from build123d import *

# Parameters (mm, degrees)
SKETCH1_R           = 9
BOSS_EXTRUDE1_DEPTH = 36
BOSS_EXTRUDE2_DEPTH = 12
SKETCH3_W           = 60
SKETCH3_H           = 72
BOSS_EXTRUDE3_DEPTH = 12
SKETCH4_W           = 13
SKETCH4_H           = 12
BOSS_EXTRUDE4_DEPTH = 60
BOSS_EXTRUDE5_DEPTH = 12


with BuildPart() as part:
    # Sketch1 → Boss-Extrude1 (new body)
    with BuildSketch(Plane.XY):
        with BuildLine():
            Line((0, -18), (60, -18))
            ThreePointArc((60, -18), (72.448153347, 13.001672133), (42.01702128, -0.782608696))
            ThreePointArc((42.01702128, -0.782608696), (40.633325006, -4.457820374), (37.021749414, -6))
            Line((37.021749414, -6), (22.978250586, -6))
            ThreePointArc((22.978250586, -6), (19.366674994, -4.457820374), (17.98297872, -0.782608696))
            ThreePointArc((17.98297872, -0.782608696), (-12.448153347, 13.001672133), (0, -18))
        make_face()
        Circle(SKETCH1_R, mode=Mode.SUBTRACT)
        with Locations((60, 0)):
            Circle(SKETCH1_R, mode=Mode.SUBTRACT)
    extrude(amount=BOSS_EXTRUDE1_DEPTH)

    # Sketch2 → Boss-Extrude2 (add)
    with BuildSketch(Plane(origin=(0, 0, 0), x_dir=(-1, 0, 0), z_dir=(0, 0, -1))):
        with BuildLine():
            Line((-60, 18), (0, 18))
            ThreePointArc((0, 18), (-13.001672133, 12.448153347), (-17.98297872, -0.782608696))
            ThreePointArc((-17.98297872, -0.782608696), (-19.366674994, -4.457820374), (-22.978250586, -6))
            Line((-22.978250586, -6), (-37.021749414, -6))
            ThreePointArc((-37.021749414, -6), (-40.633325006, -4.457820374), (-42.01702128, -0.782608696))
            ThreePointArc((-42.01702128, -0.782608696), (-46.998327867, 12.448153347), (-60, 18))
        make_face()
    extrude(amount=-BOSS_EXTRUDE2_DEPTH)

    # Sketch3 → Boss-Extrude3 (add)
    with BuildSketch(Plane(origin=(0, 0, 6), x_dir=(-1, 0, 0), z_dir=(0, 0, -1))):
        with Locations((-30, -54)):
            Rectangle(SKETCH3_W, SKETCH3_H)
        with BuildLine():
            Line((-31, -57), (-22, -57))
            ThreePointArc((-22, -57), (-14, -65), (-22, -73))
            Line((-22, -73), (-31, -73))
            ThreePointArc((-31, -73), (-39, -65), (-31, -57))
        make_face(mode=Mode.SUBTRACT)
    extrude(amount=-BOSS_EXTRUDE3_DEPTH)

    # Sketch4 → Boss-Extrude4 (add)
    with BuildSketch(Plane(origin=(60, 0, 0), x_dir=(0, 0, -1), z_dir=(1, 0, 0))):
        with Locations((0.5, -47)):
            Rectangle(SKETCH4_W, SKETCH4_H)
        with Locations((0.5, -84)):
            Rectangle(SKETCH4_W, SKETCH4_H)
    extrude(amount=-BOSS_EXTRUDE4_DEPTH)

    # Sketch5 → Boss-Extrude5 (add)
    with BuildSketch(Plane.ZY):
        Polygon((18, -90), (36, -18), (18, -18), align=None)
    extrude(amount=-BOSS_EXTRUDE5_DEPTH)


solid = part.part
Model file for the job. Use its own axes, mm. A direction names the side the tool comes from. Give positions to 0.01 mm unless a question says otherwise; leave off trailing zeros. Order: outer loops, then holes, each group sorted by start corner. A loop starts at its lowest first (then second) coordinate and runs counter-clockwise, first axis right, second up. Notation, with made-up numbers: (-10.5, 26.5) - (23.5, 26.5) arc R24 cw to (23.5, 47.5) - close; hole circle Ø4 at (73.5, 0). An arc over 180 degrees is marked (long way). Return JSON: item names as keys, results as strings.
1) Cut at A-A, the plane y = -65. Give the cut face in (x, z).
Geometry says:
{"outline": "(0, 6) - (14, 6) - (14, 18) - (12, 18) - (12, 24.25) - (0, 24.25) - close; (39, 6) - (60, 6) - (60, 18) - (39, 18) - close"}
2) Cut at C-C, the plane x = 56. Give the cut face in (y, z), plus the area to 3 significant figures.
Geometry says:
{"outline": "(-90, -7) - (-78, -7) - (-78, 6) - (-53, 6) - (-53, -7) - (-41, -7) - (-41, 6) - (-18, 6) - (-18, 0) - (-8.06, 0) - (-8.06, 36) - (-18, 36) - (-18, 18) - (-90, 18) - close; (8.06, 0) - (18, 0) - (18, 12) - (17.55, 12) - (17.55, 36) - (8.06, 36) - close", "area": "1,880 mm²"}
3) Probe line 1 (Y direction, x = 29.5, z = 3); line 2 (Y direction, x = 60, z = 25.5); line 3 (Z direction, x = 0.5, y = -12). List the from-to ranges inside material, lowest first. Write a range as from..to.
Geometry says:
{"line 1": "-90..-78, -53..-41, -18..18", "line 2": "-18..-9, 9..18", "line 3": "0..36"}
4) Pull direction X, two halves, no side cores. Call faces 1 (the flat face through (36, -18, 27)), 2 (the cylindrical face through (39, -65, 12)): pulls with the +X half, pulls with the -X half, needs draft (parallel to the pull), parting line crosses it, or undercut.
Geometry says:
{"face 1": "needs draft", "face 2": "undercut"}
5) Cut at B-B, the plane z = -3.5. Give the cut face in (x, y).
Geometry says:
{"outline": "(0, -90) - (60, -90) - (60, -78) - (0, -78) - close; (0, -53) - (60, -53) - (60, -41) - (0, -41) - close"}
6) Cut at D-D, the plane y = -4. Give the cut face in (x, z), plus the area to 3 significant figures.
Geometry says:
{"outline": "(-17.55, 0) - (-8.06, 0) - (-8.06, 36) - (-17.55, 36) - close; (8.06, 0) - (51.94, 0) - (51.94, 36) - (41.02, 36) - (41.02, 12) - (18.98, 12) - (18.98, 36) - (8.06, 36) - close; (68.06, 0) - (77.55, 0) - (77.55, 36) - (68.06, 36) - close", "area": "1,730 mm²"}
7) Flat gauge pins, fed straight in: P1, Ø3, axis at x = 46.5, y = -65.5, coming from the -Z side; P2, Ø16, axis at x = 0, y = 0, coming from the -Z side; P3, Ø8, axis at x = 39.5, z = 30, coming from the -Y side; P4, Ø7, axis at x = 33.5, z = 28, coming from the +Y side. Where does each tip first touch, or does it go through?
Geometry says:
{"P1": "z = 6", "P2": "through", "P3": "y = -18", "P4": "y = -6"}
8) 3-axis set-ups, long thin cutter, end or side, ignore diameter. For faces 3 (the flat face through (29, 0, 0)), 4 (the flat face through (30, -41, 0)), 5 (the cylindrical face through (14, -65, 12)): which of +Z, -Z, +X, -X, +Y, -Y reach the whole face in a straight line?
Geometry says:
{"face 3": "-Z, +X, -X, +Y", "face 4": "-Z, +X, -X", "face 5": "+Z, -Z"}
